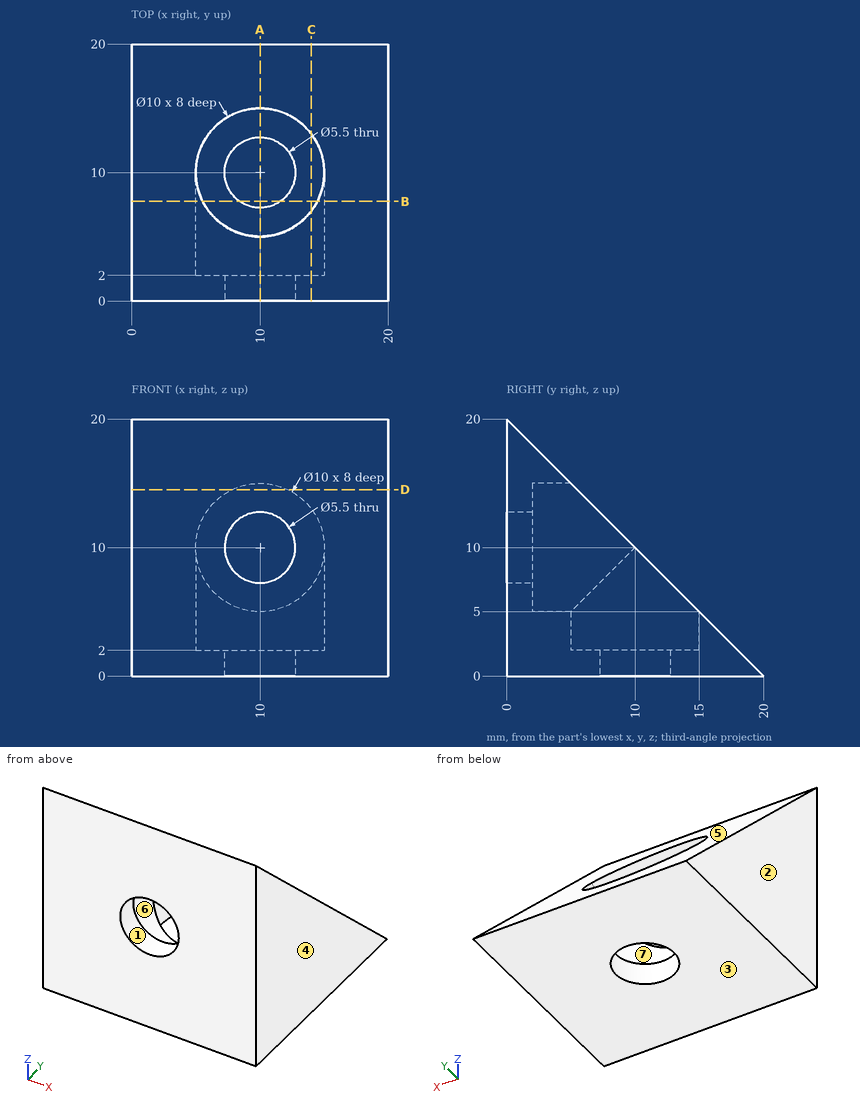
Could you check a few things on this drawing? It's one solid part, dimensions in mm from its lowest x, y, z. A direction names the side the tool comes from. Coordinates: 2 decimals unless noted, no trailing zeros. Write each loop counter-clockwise with the first axis right and the second up, starting at its lowest first coordinate (ties: lowest second). Pieces come first, ordered by that corner, then holes. Notation, with made-up numbers: (38.25, -29) - (90.25, -29) arc R19 ccw to (90.25, -16) - close; hole circle Ø8 at (-21.75, 51.5). An arc over 180 degrees is marked (long way). Use one line per item in the form item = value.
1) I need wall thicknesses on line 1 (X direction, y = 10, z = 6.25); line 2 (X direction, y = 0.6, z = 10); line 3 (Y direction, x = 16.75, z = 15). Which ranges of each line are inside material? Lowest first, please.
Solved:
line_1 = 0 to 5, 15 to 20
line_2 = 0 to 7.25, 12.75 to 20
line_3 = 0 to 5
2) On a 3-axis mill with a long thin cutter (end or side, diameter ignored), from which of +Z, -Z, +X, -X, +Y, -Y can I reach the whole of each face in a straight line? I mean the marked faces 5, 6 and 7. Say none if no direction works.
Solved:
face_5 = +Z, +X, -X, +Y
face_6 = +Y
face_7 = +Z
3) Suppose I cut it at C-C, the plane x = 14. Write out the boundary of the cut face in (y, z), plus the area to 3 significant figures.
Solved:
outline = (0, 0) - (20, 0) - (13, 7) - (13, 2) - (7, 2) - (7, 7) - (2, 7) - (2, 13) - (7, 13) - (0, 20) - close
area = 122 mm2
4) Suppose I cut it at B-B, the plane y = 7.75. Write out the boundary of the cut face in (x, z), plus the area to 3 significant figures.
Solved:
outline = (0, 0) - (8.42, 0) - (8.42, 2) - (5.53, 2) - (5.53, 7.75) arc R5 cw to (5.53, 12.25) - (0, 12.25) - close; (11.58, 0) - (20, 0) - (20, 12.25) - (14.47, 12.25) arc R5 cw to (14.47, 7.75) - (14.47, 2) - (11.58, 2) - close
area = 144 mm2
5) Suppose I cut it at D-D, the plane z = 14.5. Write out the boundary of the cut face in (x, y).
Solved:
outline = (0, 0) - (20, 0) - (20, 5.5) - (12.18, 5.5) - (12.18, 2) - (7.82, 2) - (7.82, 5.5) - (0, 5.5) - close
6) Suppose I cut it at A-A, the plane x = 10. Write out the boundary of the cut face in (y, z), plus the area to 3 significant figures.
Solved:
outline = (0, 0) - (7.25, 0) - (7.25, 2) - (5, 2) - (5, 5) - (2, 5) - (2, 7.25) - (0, 7.25) - close; (0, 12.75) - (2, 12.75) - (2, 15) - (5, 15) - (0, 20) - close; (12.75, 0) - (20, 0) - (15, 5) - (15, 2) - (12.75, 2) - close
area = 68.0 mm2
7) Thinking about a two-plate mould opening in X: for the marked faces 1, 2, 3 and 4, which applies, released by +X, released by -X, zero draft, split by the parting line, or undercut?
Solved:
face_1 = undercut
face_2 = released by -X
face_3 = zero draft
face_4 = released by +X
8) I'm going to push flat-ended pins straight in: P1, Ø6.5, axis at x = 10, z = 10, coming from the +Y side; P2, Ø2, axis at y = 14.5, z = 7, coming from the +X side (3 decimals); P3, Ø6, axis at x = 17, y = 8.5, coming from the +Z side; P4, Ø3, axis at x = 8.5, y = 12, coming from the +Z side. Where does each tip first touch, or does it pass through?
Solved:
P1 = 2
P2 = through
P3 = 14.5
P4 = 2
